Answer from the drawing. Dimensions are ordinates in mm from the lowest x, y and z of the part. Give positions to 0.01 mm unless a question says otherwise; leave off trailing zeros. Write each loop counter-clockwise with the first axis right and the second up, starting at its lowest first coordinate (ties: lowest second). Pieces come first, ordered by that corner, then holes.
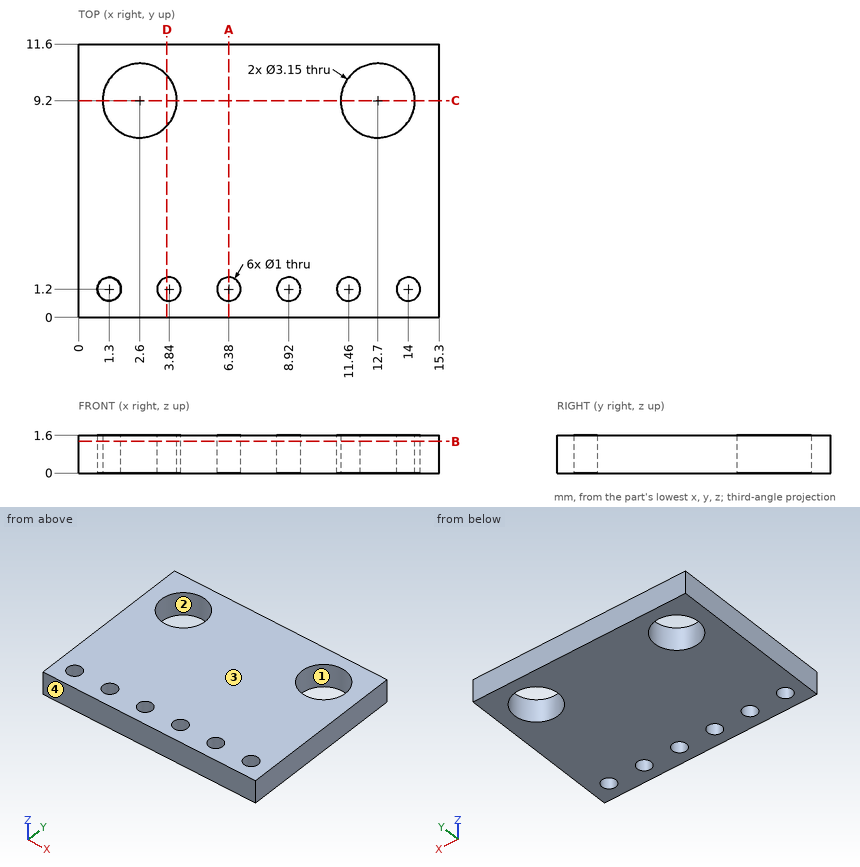
Item 1: Section B-B (z = 1.35) is taken. Give the number of separate pieces and of enclosed holes in the cut face, and give its area (3 significant figures).
Result set:
separate pieces: 1
enclosed holes: 8
area: 157 mm2
Item 2: Determine the mould class of the marked faces 1, 2, 3 and 4 for opening direction Y: pulls with the +Y half, pulls with the -Y half, needs draft (parallel to the pull), parting line crosses it, or undercut.
Result set:
face 1: undercut
face 2: undercut
face 3: needs draft
face 4: pulls with the -Y half
Item 3: Section A-A (x = 6.38) is taken. Write down the section's boundary in (y, z).
Result set:
outline: (0, 0) - (0.7, 0) - (0.7, 1.6) - (0, 1.6) - close; (1.7, 0) - (11.6, 0) - (11.6, 1.6) - (1.7, 1.6) - close
Item 4: Section D-D (x = 3.75) is taken. Write down the section's boundary in (y, z).
Result set:
outline: (0, 0) - (0.71, 0) - (0.71, 1.6) - (0, 1.6) - close; (1.69, 0) - (8.12, 0) - (8.12, 1.6) - (1.69, 1.6) - close; (10.28, 0) - (11.6, 0) - (11.6, 1.6) - (10.28, 1.6) - close
Item 5: Section C-C (y = 9.2) is taken. Write down the section's boundary in (x, z) (3 decimals).
Result set:
outline: (0, 0) - (1.025, 0) - (1.025, 1.6) - (0, 1.6) - close; (4.175, 0) - (11.125, 0) - (11.125, 1.6) - (4.175, 1.6) - close; (14.275, 0) - (15.3, 0) - (15.3, 1.6) - (14.275, 1.6) - close
Item 6: Find the intervals of material crossed by line 1 along Y through (x, z) = (3.5, 0.4); line 2 along Y through (x, z) = (1.3, 0.75); line 3 along Y through (x, z) = (8.92, 1.15), in increasing order.
Result set:
line 1: y = 0 to 0.83, 1.57 to 7.91, 10.49 to 11.6
line 2: y = 0 to 0.7, 1.7 to 8.31, 10.09 to 11.6
line 3: y = 0 to 0.7, 1.7 to 11.6
